Read the model definition and answer for the solid it produces. Units are mm, in the model's axes. Face numbers are marked on the shaded views. A direction names the side the tool comes from. Coordinates: 2 decimals unless noted, no trailing zeros. Write each loop counter-clockwise with the first axis right and the second up, starting at its lowest first coordinate (ties: lowest second). Pieces come first, ordered by that corner, then holes.
Item 1: Straight lines are drawn through the part: probe 1 along X at (y, z) = (-2, 0.25); probe 2 along Z at (x, y) = (-59, 8); probe 3 along Y at (x, z) = (24, 0.15). For each, find the intervals that lie inside material, in ascending order.
Item 2: Section D-D (x = -52) is taken. Give the vertices of the cut face in (y, z), then the cut area to 3 significant figures.
Item 3: Section A-A (z = 0.1) is taken. Give the vertices of the cut face in (x, y), then the cut area to 3 significant figures.
Item 4: This flat-tipped pin is pushed along its axis until it touches: P1, Ø3, axis at x = -19, y = -5.5, coming from the +Z side. Where does it stop, or does it pass through?
Item 5: Section B-B (y = 14.5) is taken. Give the vertices of the cut face in (x, z), then the cut area to 3 significant figures.
Item 6: A tool of negligible diameter and unlimited length cuts with its end or side. For the marked faces 1 and 2, from which of +Z, -Z, +X, -X, +Y, -Y can it reach the whole face along a straight path? Write none if from no direction.
Item 7: Section C-C (y = -6.5) is taken. Give the vertices of the cut face in (x, z), then the cut area to 3 significant figures.
Autodesk Inventor part; units mm, degrees
ref_plane "YZ Plane" through (0, 0, 0) normal (1, 0, 0) x (0, 1, 0)
ref_plane "XZ Plane" through (0, 0, 0) normal (0, 1, 0) x (-1, 0, 0)
ref_plane "XY Plane" through (0, 0, 0) normal (0, 0, 1) x (1, 0, 0)
sketch "Sketch1" plane through (0, 0, 0) normal (0, 0, 1) x (1, 0, 0)
  line L0 (-65, 12.5) -> (65, 12.5)
  line L1 (65, 12.5) -> (65, -12.5)
  line L2 (65, -12.5) -> (-65, -12.5)
  line L3 (-65, -12.5) -> (-65, 12.5)
  line L4 (-65, 12.5) -> (-65, 21.5)
  line L5 (-65, -12.5) -> (-65, -21.5)
  line L6 (65, 12.5) -> (65, 21.5)
  line L7 (65, -12.5) -> (65, -21.5)
  line L8 (-65, 21.5) -> (-40, 12.5)
  line L9 (-65, -21.5) -> (-40, -12.5)
  line L10 (40, -12.5) -> (65, -21.5)
  line L11 (40, 12.5) -> (65, 21.5)
  line L12 (65, -10.7019) -> (65, -12.5)
  line L13 (-40, 30.8502) -> (-40, -39.2706) construction
  line L14 (40, 30.8502) -> (40, -39.2706) construction
  line L15 (-122.9274, 0) -> (95.3205, 0) construction
  line L16 (0, 69.381) -> (0, -63.5203) construction
  line L17 (-65, 21.5) -> (-85, 21.5)
  line L18 (-85, 21.5) -> (-85, -21.5)
  line L19 (-85, -21.5) -> (-65, -21.5)
  line L20 (-65, -21.5) -> (-65, 21.5)
  line L21 (65, 21.5) -> (85, 21.5)
  line L22 (85, 21.5) -> (85, -21.5)
  line L23 (85, -21.5) -> (65, -21.5)
  line L24 (65, -21.5) -> (65, 21.5)
  line L25 (-65, 21.5) -> (-65, -21.5)
  point P0 (0, 0)
  point P1 (0, 0)
  point P2 (-65, 0)
  point P3 (0, 12.5)
  dimension "d0" = 130
  dimension "d1" = 25
  dimension "d2" = 40
  dimension "d3" = 40
  dimension "d4" = 20
  dimension "d5" = 20
  dimension "d15" = 43
extrude "Extrusion1" add sketch "Sketch1" along normal blind 0.2
extrude "Extrusion3" add sketch "Sketch1" along normal blind 0.4 contours L3 L5 L19 L18 L17 L4
mirror "Mirror2" about plane through (0, 0, 0) normal (1, 0, 0) of "Extrusion3"
equation "\"d11\" = material"
equation "\"d16\" = 2 * material"
properties part number "BandMiddle"
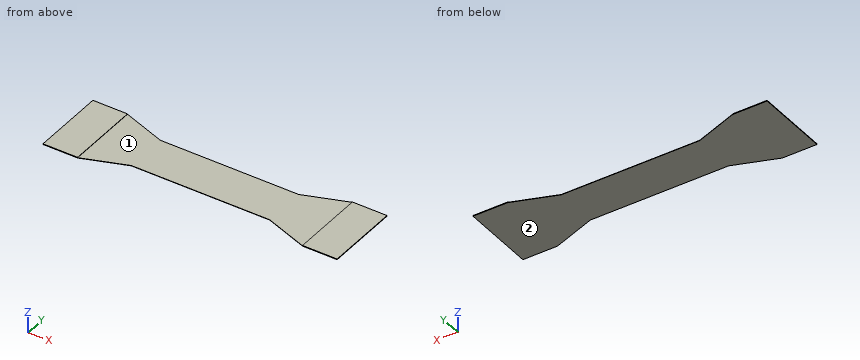
Established:
1. probe 1: x = -85 to -65, 65 to 85
1. probe 2: z = 0 to 0.2
1. probe 3: y = -12.5 to 12.5
2. outline: (-16.82, 0) - (16.82, 0) - (16.82, 0.2) - (-16.82, 0.2) - close
2. area: 6.73 mm2
3. outline: (-85, -21.5) - (-65, -21.5) - (-40, -12.5) - (40, -12.5) - (65, -21.5) - (85, -21.5) - (85, 21.5) - (65, 21.5) - (40, 12.5) - (-40, 12.5) - (-65, 21.5) - (-85, 21.5) - close
3. area: 5,420 mm2
4. P1: stops at z = 0.2
5. outline: (-85, 0) - (-45.56, 0) - (-45.56, 0.2) - (-65, 0.2) - (-65, 0.4) - (-85, 0.4) - close; (45.56, 0) - (85, 0) - (85, 0.4) - (65, 0.4) - (65, 0.2) - (45.56, 0.2) - close
5. area: 23.8 mm2
6. face 1: +Z, +Y, -Y
6. face 2: -Z, +X, -X, +Y, -Y
7. outline: (-85, 0) - (85, 0) - (85, 0.4) - (65, 0.4) - (65, 0.2) - (-65, 0.2) - (-65, 0.4) - (-85, 0.4) - close
7. area: 42.0 mm2
